Autodesk Inventor part; units mm, degrees
ref_plane "YZ Plane" through (0, 0, 0) normal (1, 0, 0) x (0, 1, 0)
ref_plane "XZ Plane" through (0, 0, 0) normal (0, 1, 0) x (-1, 0, 0)
ref_plane "XY Plane" through (0, 0, 0) normal (0, 0, 1) x (1, 0, 0)
sketch "Sketch1" plane through (0, 0, 0) normal (0, 0, 1) x (1, 0, 0)
  line L0 (-82.5, 15) -> (82.5, 15)
  line L1 (82.5, 15) -> (82.5, -15)
  line L2 (82.5, -15) -> (-82.5, -15)
  line L3 (-82.5, -15) -> (-82.5, 15)
  point P0 (0, 0)
  dimension "d0" = 165
  dimension "d1" = 30
  dimension "d2" = 82.5
  dimension "d3" = 15
extrude "Extrusion1" add sketch "Sketch1" along normal blind 10
sketch "Sketch2" plane through (0, 0, 10) normal (0, 0, 1) x (1, 0, 0)
  line L0 (82.5, 15) -> (-82.5, 15)
  point P0 (0, 0)
  point P1 (-50, 5)
  point P2 (0, 5)
  point P3 (50, 5)
  dimension "d6" = 50
  dimension "d24" = 50
  dimension "d25" = 10
hole "Hole1" at (-50, 5, 10) at (0, 5, 10) at (50, 5, 10) direction (0, 0, -1) diameter 3.4 end through all counterbore diameter 11 counterbore depth 2.6
sketch "Sketch3" plane through (0, 0, 10) normal (0, 0, 1) x (1, 0, 0)
  line L0 (82.5, 15) -> (-82.5, 15)
  circle A0 centre (0, 5) radius 1.7
  point P0 (0, 0)
  point P1 (-25, 5)
  point P2 (25, 5)
  dimension "d15" = 50
  dimension "d26" = 10
  dimension "d27" = 25
hole "Hole2" at (-25, 5, 10) at (25, 5, 10) direction (0, 0, -1) diameter 3.242 depth 11.8 tip angle 118
properties part number "zStage_jackAttach"
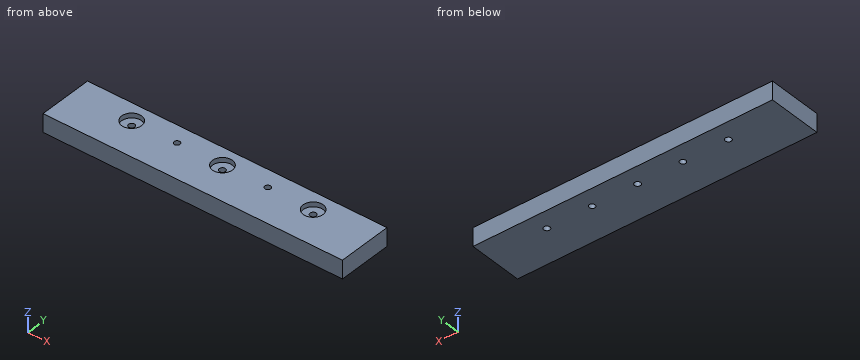
CAD build for the part. Positions are in the model's coordinates, mm. Give positions to 0.01 mm unless a question says otherwise; leave off trailing zeros. Loops run counter-clockwise (first coordinate to the right, second up) from the corner with the lowest first, then second, coordinate; pieces in that order, holes last. Notation, with made-up numbers: M -32,50.25 L 14,50.25 A21 cw 14,61.25 Z; hole C 6,16 d10. An arc over 180 degrees is marked long. Use one line per item in the form item = value.
Item 1: Slice it at C-C (x = 25). List the corners of the cut face in (y, z), plus the area to 3 significant figures.
Determined:
outline = M -15,0 L 3.38,0 L 3.38,10 L -15,10 Z; M 6.62,0 L 15,0 L 15,10 L 6.62,10 Z
area = 268 mm2
Item 2: Flat gauge pins, fed straight in: pin 1 (5.5 mm diameter, centred on x = 2.5, y = 3.5, fed in from +Z); pin 2 (4 mm diameter, centred on x = 50, y = 5, fed in from +Z). Where does each tip first touch, or does it go through?
Determined:
pin_1 = 10
pin_2 = 7.4
Item 3: Drill centre lines: probe 1 along X at (y, z) = (5, 7); probe 2 along X at (y, z) = (5, 8.2); probe 3 along Y at (x, z) = (0, 1.5). Where is each one in solid material? Low to high. Write a range as from..to.
Determined:
probe_1 = -82.5..-51.7, -48.3..-26.62, -23.38..-1.7, 1.7..23.38, 26.62..48.3, 51.7..82.5
probe_2 = -82.5..-55.5, -44.5..-26.62, -23.38..-5.5, 5.5..23.38, 26.62..44.5, 55.5..82.5
probe_3 = -15..3.3, 6.7..15
Item 4: Slice it at B-B (y = 5). Count the separate pieces of the cut face and the enclosed holes in it, plus the area to 3 significant figures.
Determined:
separate_pieces = 6
enclosed_holes = 0
area = 1,420 mm2
Item 5: Slice it at A-A (x = 0). List the corners of the cut face in (y, z), plus the area to 3 significant figures.
Determined:
outline = M -15,0 L 3.3,0 L 3.3,7.4 L -0.5,7.4 L -0.5,10 L -15,10 Z; M 6.7,0 L 15,0 L 15,10 L 10.5,10 L 10.5,7.4 L 6.7,7.4 Z
area = 246 mm2
